Geometry: final body of the model. Coordinates: model frame, mm. A direction names the side the tool comes from. Round coordinates to 2 decimals unless told otherwise and drop trailing zeros. Loops run counter-clockwise (first coordinate to the right, second up) from the corner with the lowest first, then second, coordinate; pieces in that order, holes last. Notation, with made-up numbers: (-24, 77) -> (-18, 77) arc R18 ccw to (-18, 86) -> close; hole circle Ø5 at (-4, 66.25). An arc over 180 degrees is marked (long way). Answer in a Markdown table with one row per item.
```python
from build123d import *

# Parameters (mm, degrees)
SKETCH029_W     = 3
SKETCH029_H     = 13
PAD015_DEPTH    = 2
SKETCH030_W     = 5
SKETCH030_H     = 2
SKETCH030_W_2   = 3
SKETCH030_H_2   = 0.8
SKETCH030_W_3   = 12
SKETCH030_H_3   = 2.4
PAD016_DEPTH    = 20
PAD021_DEPTH    = 2
POCKET015_DEPTH = 3
FILLET002_R     = 1
CHAMFER_SIZE    = 2
CHAMFER001_SIZE = 1.5
CHAMFER002_SIZE = 0.39


with BuildPart() as part:
    # Sketch029 → Pad015 (new body)
    with BuildSketch(Plane.XZ):
        with Locations((0.5, 4.5)):
            Rectangle(SKETCH029_W, SKETCH029_H)
    extrude(amount=PAD015_DEPTH)

    # Sketch030 (on Face6 of Pad015) → Pad016 (join)
    with BuildSketch(Plane.XZ.offset(2)):
        with Locations((-0.5, -1)):
            Rectangle(SKETCH030_W, SKETCH030_H)
        with Locations((0.5, 2.5)):
            Rectangle(SKETCH030_W_2, SKETCH030_H_2)
        with Locations((-4, 9.8)):
            Rectangle(SKETCH030_W_3, SKETCH030_H_3)
    extrude(amount=-PAD016_DEPTH)

    # Sketch036 (on Face34 of Pad016) → Pad021 (join)
    with BuildSketch(Plane(origin=(0, 0, -2), x_dir=(1, 0, 0), z_dir=(0, 0, -1))):
        Polygon((2, -18), (2, -25), (-4, -25), (-3, -18), align=None)
    extrude(amount=-PAD021_DEPTH)

    # Sketch037 (on Face35 of Pad021) → Pocket015 (cut)
    with BuildSketch(Plane(origin=(0, 0, -2), x_dir=(1, 0, 0), z_dir=(0, 0, -1))):
        with BuildLine():
            ThreePointArc((-3, -4.99), (-0.75, -2.74), (-3, -0.49))
            Line((-3, -4.99), (-3, -0.49))
        make_face()
        with BuildLine():
            ThreePointArc((-3, -18), (-0.75, -15.75), (-3, -13.5))
            Line((-3, -18), (-3, -13.5))
        make_face()
    extrude(amount=-POCKET015_DEPTH, mode=Mode.SUBTRACT)

    # Fillet002
    fillet002_edges = [part.edges().sort_by_distance(p)[0] for p in [
        (-3, 4.99, -1),
        (-3, 13.5, -1),
        (-3, 0.49, -1),
        (-3, 18, -1),
    ]]
    fillet(fillet002_edges, radius=FILLET002_R)

    # Chamfer
    chamfer_edges = [part.edges().sort_by_distance(p)[0] for p in [
        (-4, 18, 8.6),
    ]]
    chamfer(chamfer_edges, length=CHAMFER_SIZE)

    # Chamfer001
    chamfer001_edges = [part.edges().sort_by_distance(p)[0] for p in [
        (-1, 25, 0),
    ]]
    chamfer(chamfer001_edges, length=CHAMFER001_SIZE)

    # Chamfer002
    chamfer002_edges = [part.edges().sort_by_distance(p)[0] for p in [
        (0.5, 18, 2.1),
        (0.5, 18, 2.9),
    ]]
    chamfer(chamfer002_edges, length=CHAMFER002_SIZE)


with BuildPart() as part_1:
    # Body002 placement: moved
    add(part.part.moved(Location((71, -34.5, 0))))


solid = part_1.part
```
Item 1: Section query C-C, the plane x = 69.5. Output: boundary loops of the cut face in (y, z).
Ans:
| item | result |
|---|---|
| outline | (-36.5, -2) -> (-33.44, -2) -> (-33.44, 0) -> (-36.5, 0) -> close; (-36.5, 8.6) -> (-18.5, 8.6) -> (-16.5, 10.6) -> (-16.5, 11) -> (-36.5, 11) -> close; (-30.08, -2) -> (-20.43, -2) -> (-20.43, 0) -> (-30.08, 0) -> close; (-17.07, -2) -> (-9.5, -2) -> (-9.5, -1.5) -> (-11, 0) -> (-17.07, 0) -> close |
Item 2: Set-up query: faces 5 (the flat face through (61, -27, 10)), 6 (the flat face through (71, -26, 2.9)), 7 (the cylindrical face through (68.186, -21.261, -0.986)), 8 (the flat face through (70, -31.6, 2.7)), 9 (the flat face through (68, -25, -1)). Return all of +Z, -Z, +X, -X, +Y, -Y with unobstructed straight access to the full face (end or side cutting, diameter ignored); none if empty.
Ans:
| item | result |
|---|---|
| face 5 | +Z, -Z, -X, +Y, -Y |
| face 6 | +X, -X, +Y |
| face 7 | -Z, -X |
| face 8 | -X, +Y, -Y |
| face 9 | -Z, -X, -Y |
Item 3: Mould query, pull axis Z, two halves, no side actions, for faces 1 (the flat face through (67.44, -12.59, -1.01)), 2 (the flat face through (71, -26, 2.1)), 3 (the flat face through (70, -10, -1)), 4 (the flat face through (67, -28, 8.6)). Classes: released by +Z, released by -Z, zero draft, split by the parting line, or undercut.
Ans:
| item | result |
|---|---|
| face 1 | zero draft |
| face 2 | undercut |
| face 3 | released by +Z |
| face 4 | undercut |
Item 4: Ray query, L1, parallel to Z at x = 72.5, y = -22.5; L2, parallel to Z at x = 69.25, y = -26.75; L3, parallel to Z at x = 63.75, y = -21.5. Return the intervals inside material, ascending.
Ans:
| item | result |
|---|---|
| L1 | -2 to 0, 2.1 to 2.9, 8.6 to 11 |
| L2 | -2 to 0, 8.6 to 11 |
| L3 | 8.6 to 11 |
Item 5: First-contact query: P1, Ø6, axis at x = 65.5, y = -31, coming from the -Z side; P2, Ø1.5, axis at x = 72, z = 6.5, coming from the +Y side; P3, Ø4.5, axis at y = -22, z = 3, coming from the -X side; P4, Ø1, axis at x = 65.5, z = 1, coming from the -Y side. Flat tips, straight axial feed; report the tip coordinate or a pass-through.
Ans:
| item | result |
|---|---|
| P1 | z = 8.6 |
| P2 | y = -34.5 |
| P3 | x = 70 |
| P4 | through |
Item 6: Section query D-D, the plane y = -33.25. Output: boundary loops of the cut face in (x, z), and give its area (3 significant figures).
Ans:
| item | result |
|---|---|
| outline | (61, 8.6) -> (73, 8.6) -> (73, 11) -> (61, 11) -> close; (69.69, -2) -> (73, -2) -> (73, 0) -> (69.69, 0) -> close; (70, 2.1) -> (73, 2.1) -> (73, 2.9) -> (70, 2.9) -> close |
| area | 37.8 mm2 |
Item 7: Section query A-A, the plane y = -25.5. Output: boundary loops of the cut face in (x, z), and give its area (3 significant figures).
Ans:
| item | result |
|---|---|
| outline | (61, 8.6) -> (73, 8.6) -> (73, 11) -> (61, 11) -> close; (68, -2) -> (73, -2) -> (73, 0) -> (68, 0) -> close; (70, 2.1) -> (73, 2.1) -> (73, 2.9) -> (70, 2.9) -> close |
| area | 41.2 mm2 |
